from build123d import *

# Parameters (mm, degrees)
F0_W     = 101.6
F0_H     = 101.6
F1_DEPTH = 38.1
F4_DEPTH = 50.8
F5_ANGLE = 70
F6_DEPTH = 50.8


with BuildPart() as f1:
    # F0 (on Top) → F1 (new body, symmetric)
    with BuildSketch(Plane.XY):
        Rectangle(F0_W, F0_H)
    extrude(amount=F1_DEPTH, both=True)

    # F3 (on Right) → F4 (cut, symmetric)
    with BuildSketch(Plane.YZ):
        with BuildLine():
            Line((0, -25.4), (0, -38.1))
            Line((0, -38.1), (50.8, -38.1))
            Line((50.8, -38.1), (50.8, 0))
            Line((50.8, 0), (25.4, 0))
            ThreePointArc((25.4, 0), (7.439488, -7.439488), (0, -25.4))
        make_face()
    extrude(amount=F4_DEPTH, both=True, mode=Mode.SUBTRACT)

    # F3 (on Right) → F5 (revolve, symmetric, cut)
    with BuildSketch(Plane.YZ) as f5_sk:
        with BuildLine():
            ThreePointArc((-43.385721, -38.1), (-50.8, 0), (-43.385721, 38.1))
            Line((-43.385721, 38.1), (-68.785721, 38.1))
            Line((-68.785721, 38.1), (-68.785721, -38.1))
            Line((-68.785721, -38.1), (-43.385721, -38.1))
        make_face()
    revolve(axis=Axis((0, 50.8, 0), (0, 0, -1)), revolution_arc=F5_ANGLE / 2, mode=Mode.SUBTRACT)
    revolve(f5_sk.sketch, axis=Axis((0, 50.8, 0), (0, 0, 1)), revolution_arc=F5_ANGLE / 2, mode=Mode.SUBTRACT)

    # F3 (on Right) → F6 (join, symmetric)
    with BuildSketch(Plane.YZ):
        with BuildLine():
            Line((50.8, 38.1), (50.8, 0))
            ThreePointArc((50.8, 0), (57.15, 19.05), (50.8, 38.1))
        make_face()
    extrude(amount=F6_DEPTH, both=True)


solid = f1.part
Verification items for the finished model (mm, model axes). A direction names the side the tool comes from. Give positions to 0.01 mm unless a question says otherwise; leave off trailing zeros. Loops run counter-clockwise (first coordinate to the right, second up) from the corner with the lowest first, then second, coordinate; pieces in that order, holes last.
1) Sectioned sample at A-A, the plane y = 33. Enter the section's corners in (x, z).
2) Thickness scan on line 1 along Z through (x, y) = (-38.5, 39); line 2 along Z through (x, y) = (-6, 21); line 3 along Y through (x, z) = (33, 16.5). Record the ranges inside material, lowest first.
3) Sectioned sample at B-B, the plane y = 6. Enter the section's corners in (x, z).
4) Set-up check for faces 1 (the cylindrical face through (0.71, 57.15, 18.76)), 2 (the flat face through (1, 0, -32)): record each of +Z, -Z, +X, -X, +Y, -Y from which the full face is reachable in a straight line by a thin tool's end or side.
5) Depth check by flat-ended pin: pin 1 Ø5 at (x, z) = (9, -28.5) entering from +Y; pin 2 Ø1.5 at (x, z) = (-12, -16) entering from +Y; pin 3 Ø2 at (x, y) = (31.5, 31.5) entering from -Z. Enter the tip coordinate at first touch or a pass-through.
Answers:
1. outline: (-50.8, 0) - (50.8, 0) - (50.8, 38.1) - (-50.8, 38.1) - close
2. line 1: z = 0 to 38.1
2. line 2: z = -0.38 to 38.1
2. line 3: y = -43.86 to 57.05
3. outline: (-50.8, -9) - (50.8, -9) - (50.8, 38.1) - (-50.8, 38.1) - close
4. face 1: +X, -X, +Y
4. face 2: -Z, +X, -X, +Y
5. pin 1: stops at y = 0
5. pin 2: stops at y = 2.12
5. pin 3: stops at z = 0
